Work out the finished part from the listing and answer in its coordinate system (mm). A direction names the side the tool comes from. Coordinates: 2 decimals unless noted, no trailing zeros. Order: outer loops, then holes, each group sorted by start corner. A loop starts at its lowest first (then second) coordinate and runs counter-clockwise, first axis right, second up. Notation, with made-up numbers: (47.5, -38) - (52.5, -38) arc R4 ccw to (52.5, -33) - close; hole circle Ø5 at (39.25, -18). An arc over 180 degrees is marked (long way). Answer as a JSON object with one key per item and string values. Group by question number.
1) Section A-A (x = 54) is taken. Give the vertices of the cut face in (y, z).
2) Section B-B (z = 43.5) is taken. Give the vertices of the cut face in (x, y), plus the area to 3 significant figures.
3) Section D-D (x = -32) is taken. Give the vertices of the cut face in (y, z), plus the area to 3 significant figures.
4) The mould has two halves that part along Y. Classify faces 4 (the face through (58, 31, 12.7)), 5 (the face through (0.7, -6.4, 44.5)), 6 (the face through (-1, 38.1, 31)), 7 (the face through (-1, -38.1, 31)): released by +Y, released by -Y, zero draft, split by the parting line, or undercut.
5) A tool of negligible diameter and unlimited length cuts with its end or side. For faces 1 (the face through (-1, -1, 19.05)), 2 (the face through (-50.8, -1, 32)), 3 (the face through (58, -31, 12.7)), from which of +Z, -Z, +X, -X, +Y, -Y can it reach the whole face along a straight path? Write none if from no direction.
6) Each of these flat-tipped pins is pushed along its axis until it touches: P1, Ø5, axis at y = 18.5, z = 23, coming from the -X side; P2, Ø4, axis at x = -1, y = -6.5, coming from the +Z side; P3, Ø12.5, axis at x = 65, y = -26.5, coming from the +Z side. Where does it stop, or does it pass through?
7) Section C-C (y = 5) is taken. Give the vertices of the cut face in (x, z), plus the area to 3 significant figures.
8) Find the intervals of material crossed by line 1 along X through (y, z) = (-1.5, 7); line 2 along Z through (x, y) = (-8.5, -28); line 3 along X through (y, z) = (23, 44), in increasing order.
from build123d import *

# Parameters (mm, degrees)
F1_DEPTH = 38.1
F3_DEPTH = 12.701
F5_DEPTH = 127.001


with BuildPart() as f1:
    # F0 (on Front) → F1 (new body, symmetric)
    with BuildSketch(Plane.XZ):
        Polygon((-38.1, 19.05), (0, 19.05), (38.1, 19.05), (38.1, 0), (76.2, 0), (76.2, 12.7), (50.8, 12.7), (50.8, 50.8), (-50.8, 50.8), (-50.8, 12.7), (-76.2, 12.7), (-76.2, 0), (-38.1, 0), align=None)
    extrude(amount=F1_DEPTH, both=True)

    # F2 (on face) → F3 (cut, through all)
    with BuildSketch(Plane.XY.offset(12.7)):
        Polygon((50.8, -12.7), (76.2, -38.1), (76.2, 38.1), (50.8, 12.7), align=None)
    extrude(amount=-F3_DEPTH, mode=Mode.SUBTRACT)

    # F4 (on face) → F5 (cut, through all)
    with BuildSketch(Plane.YZ.offset(50.8)):
        Polygon((12.7, 50.8), (-12.7, 50.8), (0, 38.1), align=None)
    extrude(amount=-F5_DEPTH, mode=Mode.SUBTRACT)


solid = f1.part
Report:
{
 "1": {"outline": "(-38.1, 0) - (-15.9, 0) - (-15.9, 12.7) - (-38.1, 12.7) - close; (15.9, 0) - (38.1, 0) - (38.1, 12.7) - (15.9, 12.7) - close"},
 "2": {"outline": "(-50.8, -38.1) - (50.8, -38.1) - (50.8, -5.4) - (-50.8, -5.4) - close; (-50.8, 5.4) - (50.8, 5.4) - (50.8, 38.1) - (-50.8, 38.1) - close", "area": "6,640 mm²"},
 "3": {"outline": "(-38.1, 19.05) - (38.1, 19.05) - (38.1, 50.8) - (12.7, 50.8) - (0, 38.1) - (-12.7, 50.8) - (-38.1, 50.8) - close", "area": "2,260 mm²"},
 "4": {"face 4": "zero draft", "face 5": "undercut", "face 6": "released by +Y", "face 7": "released by -Y"},
 "5": {"face 1": "-Z, +Y, -Y", "face 2": "+Z, -X, +Y, -Y", "face 3": "+Z, +X, +Y, -Y"},
 "6": {"P1": "stops at x = -50.8", "P2": "stops at z = 46.6", "P3": "stops at z = 12.7"},
 "7": {"outline": "(-76.2, 0) - (-38.1, 0) - (-38.1, 19.05) - (38.1, 19.05) - (38.1, 0) - (50.8, 0) - (50.8, 43.1) - (-50.8, 43.1) - (-50.8, 12.7) - (-76.2, 12.7) - close", "area": "3,250 mm²"},
 "8": {"line 1": "x = -76.2 to -38.1, 38.1 to 50.8", "line 2": "z = 19.05 to 50.8", "line 3": "x = -50.8 to 50.8"}
}
